from build123d import *

# Parameters (mm, degrees)
F1_DEPTH = 3.175


with BuildPart() as f1:
    # F0 (on Top) → F1 (new body)
    with BuildSketch(Plane.XY):
        with BuildLine():
            Line((-19.06356, 1.432344), (-19.06356, -4.567656))
            Line((-19.06356, -4.567656), (-4.276681, -4.567656))
            Line((-4.276681, -4.567656), (-4.276681, -7.742656))
            Line((-4.276681, -7.742656), (5.723319, -7.742656))
            Line((5.723319, -7.742656), (5.723319, -4.567656))
            Line((5.723319, -4.567656), (20.510198, -4.567656))
            Line((20.510198, -4.567656), (20.510198, 1.432344))
            ThreePointArc((20.510198, 1.432344), (0.723319, 21.219223), (-19.06356, 1.432344))
        make_face()
        with BuildLine():
            Line((9.655452, 0.432344), (5.723319, 0.432344))
            Line((5.723319, 0.432344), (-4.276681, 0.432344))
            Line((-4.276681, 0.432344), (-8.208814, 0.432344))
            ThreePointArc((-8.208814, 0.432344), (-12.405108, 2.713683), (-12.772135, 7.475896))
            ThreePointArc((-12.772135, 7.475896), (0.723319, 16.219223), (14.218773, 7.475896))
            ThreePointArc((14.218773, 7.475896), (13.851746, 2.713683), (9.655452, 0.432344))
        make_face(mode=Mode.SUBTRACT)
    extrude(amount=F1_DEPTH)


solid = f1.part
Could you check a few things on this model? Use its own coordinates, in mm. A direction names the side the tool comes from. Give positions to 0.01 mm unless a question says otherwise; leave off trailing zeros. Order: outer loops, then holes, each group sorted by start corner. A loop starts at its lowest first (then second) coordinate and runs counter-clockwise, first axis right, second up. Notation, with made-up numbers: (-22.5, 64.25) -> (24.5, 64.25) arc R34 ccw to (24.5, 102.25) -> close; hole circle Ø7 at (81, 42.25). An arc over 180 degrees is marked (long way). Return JSON: item names as keys, results as strings.
1. Thinking about a two-plate mould opening in Y: for faces 5 (the cylindrical face through (0.485, 16.217, 1.565)), 6 (the flat face through (5.723, -6, 2)), 7 (the flat face through (-12, -4.568, 2)), which applies, pulls with the +Y half, pulls with the -Y half, needs draft (parallel to the pull), parting line crosses it, or undercut?
Answer list:
{"face 5": "undercut", "face 6": "needs draft", "face 7": "pulls with the -Y half"}
2. I need wall thicknesses on line 1 (Y direction, x = -7.5, z = 2.8); line 2 (Y direction, x = 14, z = 0.8); line 3 (X direction, y = 2, z = 0.9). Which ranges of each line are inside material? Lowest first, please. Write a range as from..to.
Answer list:
{"line 1": "y = -4.57..0.43, 13.72..19.43", "line 2": "y = -4.57..2.96, 7.94..16.1", "line 3": "x = -19.06..-11.84, 13.29..20.5"}
3. On a 3-axis mill with a long thin cutter (end or side, diameter ignored), from which of +Z, -Z, +X, -X, +Y, -Y can I reach the whole of each face in a straight line? I mean faces 1 (the flat face through (1, 0.432, 2)), 2 (the flat face through (13, -4.568, 2)), 3 (the flat face through (0, -3, 0)), 4 (the flat face through (-4.277, -6, 2)). Say none if no direction works.
Answer list:
{"face 1": "+Z, -Z", "face 2": "+Z, -Z, +X, -Y", "face 3": "-Z, +X, -X, +Y, -Y", "face 4": "+Z, -Z, -X, -Y"}
4. Imagine slicing it at C-C on x = -9.5. List the corners of the cut face in (y, z) for me (3 decimals), then the cut area to 3 significant figures.
Answer list:
{"outline": "(-4.568, 0) -> (0.602, 0) -> (0.602, 3.175) -> (-4.568, 3.175) -> close; (12.116, 0) -> (18.374, 0) -> (18.374, 3.175) -> (12.116, 3.175) -> close", "area": "36.3 mm2"}
5. Imagine slicing it at D-D on y = -5. List the corners of the cut face in (x, z) for me (3 decimals), then the cut area to 4 significant figures.
Answer list:
{"outline": "(-4.277, 0) -> (5.723, 0) -> (5.723, 3.175) -> (-4.277, 3.175) -> close", "area": "31.75 mm2"}
6. Imagine slicing it at B-B on y = 6.5. List the corners of the cut face in (x, z) for me (1 decimal).
Answer list:
{"outline": "(-18.4, 0) -> (-13.1, 0) -> (-13.1, 3.2) -> (-18.4, 3.2) -> close; (14.5, 0) -> (19.9, 0) -> (19.9, 3.2) -> (14.5, 3.2) -> close"}
7. For pin 1 Ø1.6 at (y, z) = (-6.5, 1.5) entering from -X; pin 2 Ø1 at (y, z) = (-6, 1) entering from +X; pin 3 Ø1.6 at (x, z) = (3.5, 1.5) entering from +Y, each with a flat end and sliding along its axis, tell me the tip position at first contact or that it passes through.
Answer list:
{"pin 1": "stops at x = -4.28", "pin 2": "stops at x = 5.72", "pin 3": "stops at y = 21.12"}
